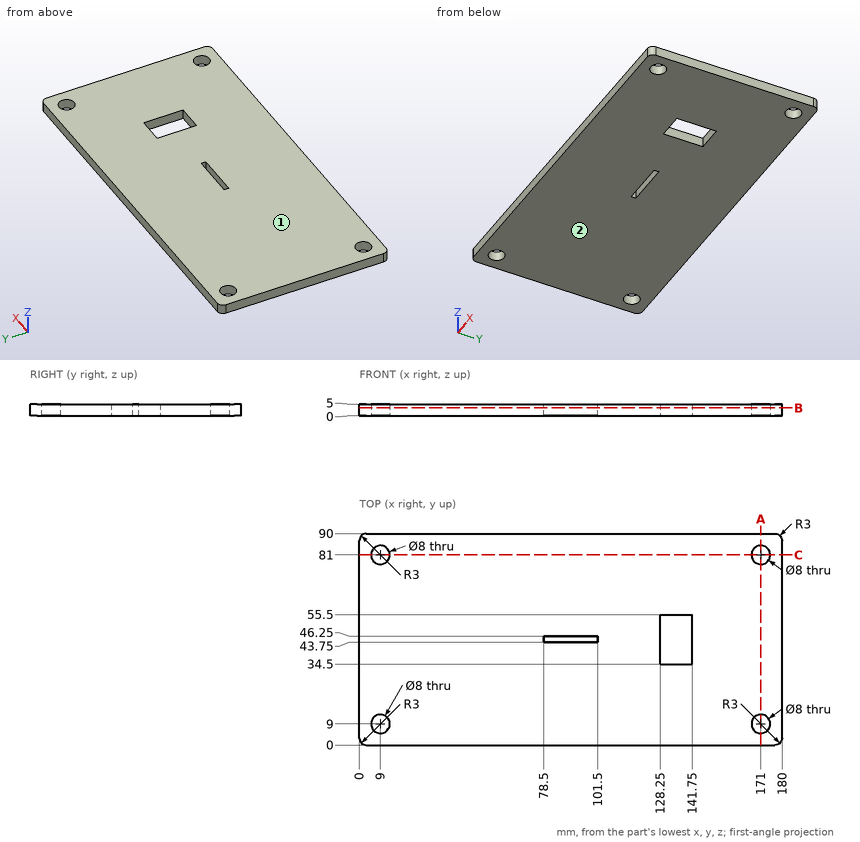
Here's the drawing with two shaded views (mm, measured from the low corner). I have some questions. Give positions to 0.01 mm unless a question says otherwise; leave off trailing zeros. Order: outer loops, then holes, each group sorted by start corner. A loop starts at its lowest first (then second) coordinate and runs counter-clockwise, first axis right, second up. Notation, with made-up numbers: (-19, 4.5) - (26, 4.5) arc R14 ccw to (26, 19.5) - close; hole circle Ø4 at (-39, -32). An arc over 180 degrees is marked (long way). Write each question's results on one line, items separated by ' | '.
1) Suppose I cut it at B-B, the plane z = 3.4. Write out the boundary of the cut face in (x, y).
Final values:
outline: (0, 3) arc R3 ccw to (3, 0) - (177, 0) arc R3 ccw to (180, 3) - (180, 87) arc R3 ccw to (177, 90) - (3, 90) arc R3 ccw to (0, 87) - close; hole circle Ø8 at (9, 9); hole circle Ø8 at (9, 81); hole (78.5, 43.75) - (101.5, 43.75) - (101.5, 46.25) - (78.5, 46.25) - close; hole (128.25, 34.5) - (141.75, 34.5) - (141.75, 55.5) - (128.25, 55.5) - close; hole circle Ø8 at (171, 9); hole circle Ø8 at (171, 81)
2) I'm going to push a flat-ended pin straight in: pin 1 Ø7 at (x, y) = (171, 81) entering from -Z. Where does the tip first touch, or does it pass through?
Final values:
pin 1: passes through
3) Please list where these lines run through material, in increasing order: line 1 along Y through (x, z) = (171, 1); line 2 along Y through (x, z) = (138, 4.35); line 3 along X through (y, z) = (42.5, 1.75). Write a range as [from, to].
Final values:
line 1: y = [0, 5], [13, 77], [85, 90] | line 2: y = [0, 34.5], [55.5, 90] | line 3: x = [0, 128.25], [141.75, 180]
4) Suppose I cut it at A-A, the plane x = 171. Write out the boundary of the cut face in (y, z).
Final values:
outline: (0, 0) - (5, 0) - (5, 5) - (0, 5) - close; (13, 0) - (77, 0) - (77, 5) - (13, 5) - close; (85, 0) - (90, 0) - (90, 5) - (85, 5) - close
5) Suppose I cut it at C-C, the plane y = 81. Write out the boundary of the cut face in (x, z).
Final values:
outline: (0, 0) - (5, 0) - (5, 5) - (0, 5) - close; (13, 0) - (167, 0) - (167, 5) - (13, 5) - close; (175, 0) - (180, 0) - (180, 5) - (175, 5) - close
6) If we mould it in two halves opening along Z, with no side actions, what happens to the marked faces 1 and 2? For each: pulls with the +Z half, pulls with the -Z half, needs draft (parallel to the pull), parting line crosses it, or undercut.
Final values:
face 1: pulls with the +Z half | face 2: pulls with the -Z half
